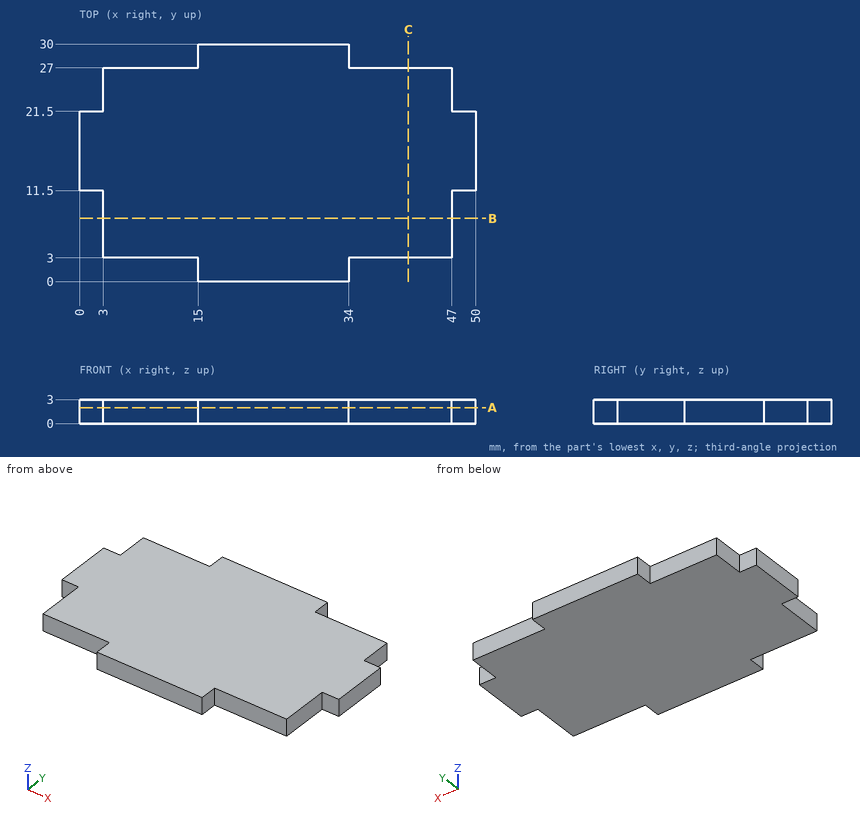
Could you check a few things on this drawing? It's one solid part, dimensions in mm from its lowest x, y, z. Coordinates: 2 decimals unless noted, no trailing zeros. Order: outer loops, then holes, each group sorted by start corner. A loop starts at its lowest first (then second) coordinate and runs counter-clockwise, first axis right, second up. Notation, with made-up numbers: (13, 63) -> (68, 63) arc R23 ccw to (68, 79) -> close; hole circle Ø2 at (-23.5, -7). An arc over 180 degrees is marked (long way). Answer in a Markdown table with one row per item.
(1) Will these pins go through, and if not, where does the flat tip stop? pin 1 Ø1.5 at (y, z) = (5.5, 1.5) entering from +X; pin 2 Ø0.9 at (x, z) = (40.5, 1.5) entering from -Y; pin 3 Ø1 at (x, z) = (5.5, 1.5) entering from +Y.
Answer key:
| item | result |
|---|---|
| pin 1 | x = 47 |
| pin 2 | y = 3 |
| pin 3 | y = 27 |
(2) I want a section at A-A on z = 2. List the corners of the cut face in (x, y) for me.
Answer key:
| item | result |
|---|---|
| outline | (0, 11.5) -> (3, 11.5) -> (3, 3) -> (15, 3) -> (15, 0) -> (34, 0) -> (34, 3) -> (47, 3) -> (47, 11.5) -> (50, 11.5) -> (50, 21.5) -> (47, 21.5) -> (47, 27) -> (34, 27) -> (34, 30) -> (15, 30) -> (15, 27) -> (3, 27) -> (3, 21.5) -> (0, 21.5) -> close |
(3) I want a section at B-B on y = 8. List the corners of the cut face in (x, z) for me, then the cut area to 3 significant figures.
Answer key:
| item | result |
|---|---|
| outline | (3, 0) -> (47, 0) -> (47, 3) -> (3, 3) -> close |
| area | 132 mm^2 |
(4) Please list where these lines run through material, in increasing order: probe 1 along X at (y, z) = (25, 2.8); probe 2 along Y at (x, z) = (38, 1.1); probe 3 along X at (y, z) = (28.25, 2.6).
Answer key:
| item | result |
|---|---|
| probe 1 | 3 to 47 |
| probe 2 | 3 to 27 |
| probe 3 | 15 to 34 |
(5) I want a section at C-C on x = 41.5. List the corners of the cut face in (y, z) for me, then the cut area to 3 significant figures.
Answer key:
| item | result |
|---|---|
| outline | (3, 0) -> (27, 0) -> (27, 3) -> (3, 3) -> close |
| area | 72.0 mm^2 |
